Geometry: final body of the model. Coordinates: model frame, mm. Face numbers are marked on the shaded views. Coordinates: 2 decimals unless noted, no trailing zeros. Loops run counter-clockwise (first coordinate to the right, second up) from the corner with the lowest first, then second, coordinate; pieces in that order, holes last. Notation, with made-up numbers: (37.5, 18.25) - (63.5, 18.25) arc R34 ccw to (63.5, 49.25) - close; hole circle Ø5 at (-33.5, 13.25). An arc over 180 degrees is marked (long way). Answer in a Markdown table with one row per item.
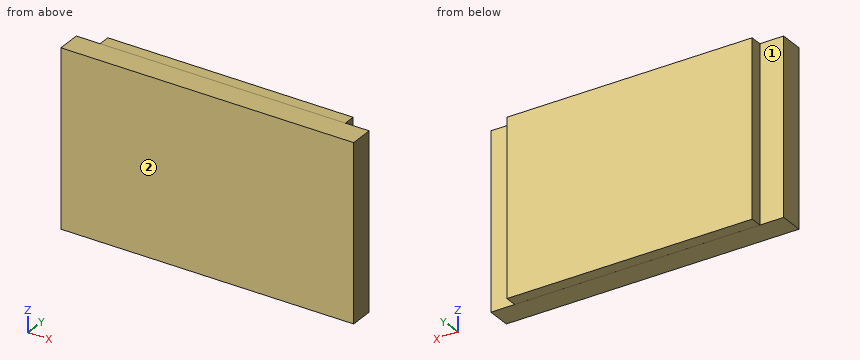
from build123d import *

# Parameters (mm, degrees)
BOSS_EXTRUDE1_START = 2
SKETCH1_W           = 41.337660338
SKETCH1_H           = 29.52690024
BOSS_EXTRUDE1_DEPTH = 2
BOSS_EXTRUDE2_START = -2
SKETCH2_W           = 49.34
SKETCH2_H           = 29.53
BOSS_EXTRUDE2_DEPTH = 4


with BuildPart() as part:
    # Sketch1 → Boss-Extrude1 (new body)
    with BuildSketch(Plane(origin=(0, 0, 0), x_dir=(1, 0, 0), z_dir=(0, 1, 0)).offset(BOSS_EXTRUDE1_START)):
        Rectangle(SKETCH1_W, SKETCH1_H)
    extrude(amount=BOSS_EXTRUDE1_DEPTH)

    # Sketch2 → Boss-Extrude2 (add)
    with BuildSketch(Plane(origin=(0, 0, 0), x_dir=(1, 0, 0), z_dir=(0, 1, 0)).offset(BOSS_EXTRUDE2_START)):
        Rectangle(SKETCH2_W, SKETCH2_H)
    extrude(amount=BOSS_EXTRUDE2_DEPTH)


solid = part.part
(1) Cut plane B-B on y = 3.5. Output: boundary loops of the cut face in (x, z), then the cut area to 3 significant figures.
Verdict:
| item | result |
|---|---|
| outline | (-20.67, -14.76) - (20.67, -14.76) - (20.67, 14.76) - (-20.67, 14.76) - close |
| area | 1,220 mm² |
(2) First-contact query: pin 1 Ø2 at (y, z) = (3.5, 7) entering from +X. Flat tip, straight axial feed; report the tip coordinate or a pass-through.
Verdict:
| item | result |
|---|---|
| pin 1 | stops at x = 20.67 |
(3) Ray query, probe 1 along Z at (x, y) = (14.5, 2); probe 2 along X at (y, z) = (3.1, 0.5). Return the intervals inside material, ascending.
Verdict:
| item | result |
|---|---|
| probe 1 | z = -14.76 to 14.76 |
| probe 2 | x = -20.67 to 20.67 |
(4) Pull-direction query (Y, two-part tool) for the marked faces 1 and 2; classes: pulls with the +Y half, pulls with the -Y half, needs draft (parallel to the pull), parting line crosses it, or undercut.
Verdict:
| item | result |
|---|---|
| face 1 | pulls with the +Y half |
| face 2 | pulls with the -Y half |
(5) Cut plane A-A on z = 2.5. Output: boundary loops of the cut face in (x, y).
Verdict:
| item | result |
|---|---|
| outline | (-24.67, -2) - (24.67, -2) - (24.67, 2) - (20.67, 2) - (20.67, 4) - (-20.67, 4) - (-20.67, 2) - (-24.67, 2) - close |
